Answer from the drawing. Dimensions are ordinates in mm from the lowest x, y and z of the part. Coordinates: 2 decimals unless noted, no trailing zeros. Write each loop counter-clockwise with the first axis right and the second up, starting at its lowest first coordinate (ties: lowest second). Pieces come first, ordered by that corner, then holes. Notation, with made-up numbers: (19, -9) -> (68, -9) arc R25 ccw to (68, 18) -> close; hole circle Ø1 at (37.25, 33). An arc over 180 degrees is marked (long way). One line per item, written item: value. Start each with the question number.
1. Find section B-B, the plane z = 41. Write down the section's boundary in (x, y), and give its area (3 significant figures).
2. Given P1, Ø8, axis at x = 34, y = 59.5, coming from the +Z side; P2, Ø3, axis at x = 46, z = 98.5, coming from the +Y side; P3, Ø5, axis at x = 53, z = 100, coming from the +Y side, each flat-ended and moving along its own axis, determine where each tip first touches the part or whether it passes through.
3. Consider line 1 along X through (y, z) = (40, 83); line 2 along X through (y, z) = (21.5, 85.5). Determine where each line is inside the solid, lowest interval first.
4. For a pull along X with two mould halves and no side action, classify the marked faces 1, 2 and 3 as pulls with the +X half, pulls with the -X half, needs draft (parallel to the pull), parting line crosses it, or undercut.
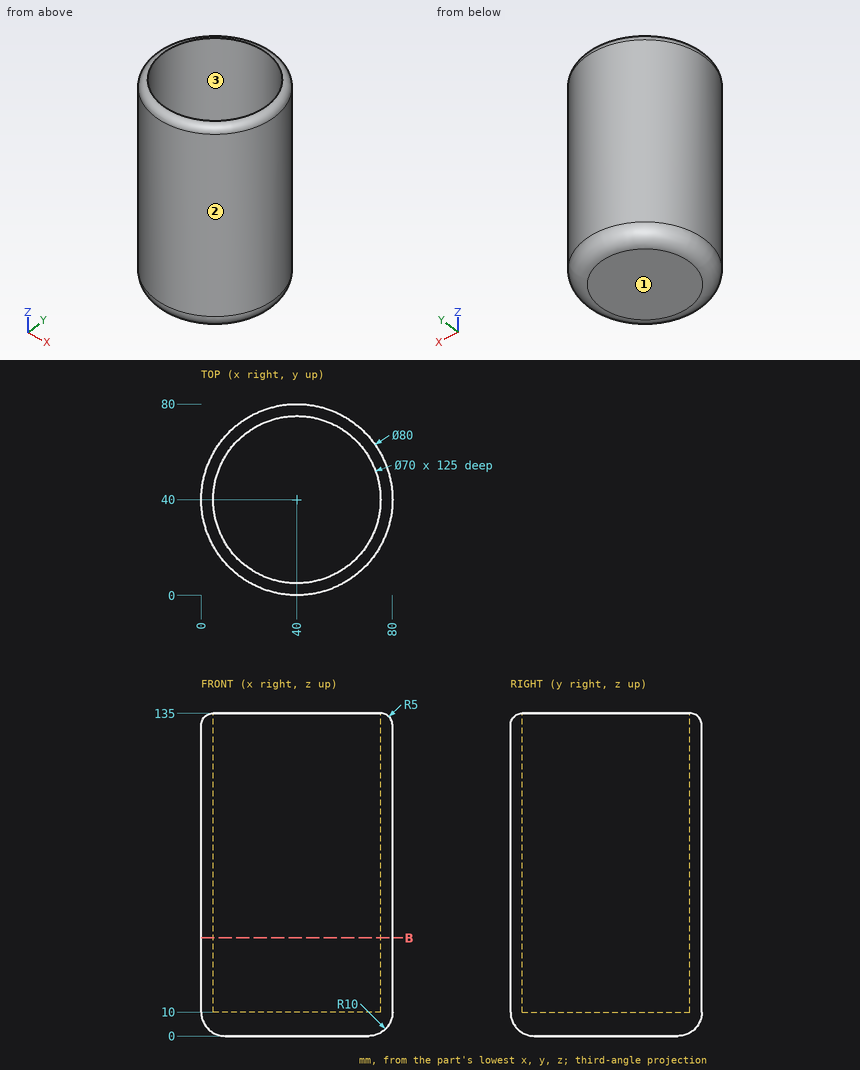
Answer block:
1. outline: circle Ø80 at (40, 40); hole circle Ø70 at (40, 40)
1. area: 1,180 mm2
2. P1: stops at z = 10
2. P2: stops at y = 79.75
2. P3: stops at y = 78.6
3. line 1: x = 0 to 5, 75 to 80
3. line 2: x = 4.54 to 10.29, 69.71 to 75.46
4. face 1: needs draft
4. face 2: parting line crosses it
4. face 3: undercut
